Here's how the part is built. I have some questions about the finished solid (model axes, mm). Give positions to 0.01 mm unless a question says otherwise; leave off trailing zeros. Order: outer loops, then holes, each group sorted by start corner. A loop starts at its lowest first (then second) coordinate and runs counter-clockwise, first axis right, second up. Notation, with made-up numbers: (67.5, 44.25) - (126.5, 44.25) arc R11 ccw to (126.5, 63.25) - close; hole circle Ø9 at (-4, -5). An arc over 180 degrees is marked (long way). One line per question, with ' | ' between items.
Autodesk Inventor part; units mm, degrees
ref_plane "YZ Plane" through (0, 0, 0) normal (1, 0, 0) x (0, 1, 0)
ref_plane "XZ Plane" through (0, 0, 0) normal (0, 1, 0) x (-1, 0, 0)
ref_plane "XY Plane" through (0, 0, 0) normal (0, 0, 1) x (1, 0, 0)
sketch "スケッチ1" plane through (0, 0, 0) normal (0, 1, 0) x (-1, 0, 0)
  line L0 (0, 0) -> (-287.5, 0)
  line L1 (-287.5, 0) -> (-287.5, -30)
  line L2 (-287.5, -30) -> (0, -30)
  line L3 (0, -30) -> (0, 0)
  arc A0 (-17.5, -30) -> (-17.5, 0) centre (-17.5, -15) ccw
  point P0 (-17.5, -12.5)
  dimension "d0" = 287.5
  dimension "d1" = 30
  dimension "d2" = 17.5
  dimension "d3" = 17.5
  dimension "d43" = 17.5
extrude "押し出し1" add sketch "スケッチ1" along normal blind 3 contours A0 L2 L1 L0
sketch "スケッチ2" plane through (0, 3, 0) normal (0, 1, 0) x (1, 0, 0)
  arc A0 (17.5, 30) -> (17.5, 0) centre (17.5, 15) ccw
  line L0 (287.5, 30) -> (17.5, 30)
  point P0 (0, 0)
  point P1 (2.5, 15)
hole "穴1" at (17.5, 3, -15) direction (0, -1, 0) diameter 16 end through all
sketch "スケッチ3" plane through (0, 3, 0) normal (0, 1, 0) x (1, 0, 0)
  line L0 (287.5, 0) -> (287.5, 30)
  arc A0 (17.5, 30) -> (17.5, 0) centre (17.5, 15) ccw construction
  line L1 (17.5, 15) -> (287.5, 15) construction
  line L2 (287.5, 0) -> (287.5, 30) construction
  point P0 (0, 0)
  point P1 (57.5, 15)
  point P2 (67.5, 15)
  point P3 (77.5, 15)
  point P4 (87.5, 15)
  point P5 (97.5, 15)
  point P6 (107.5, 15)
  point P7 (117.5, 15)
  point P8 (127.5, 15)
  point P9 (137.5, 15)
  point P10 (147.5, 15)
  point P11 (157.5, 15)
  point P12 (167.5, 15)
  point P13 (177.5, 15)
  point P14 (187.5, 15)
  point P15 (197.5, 15)
  point P16 (207.5, 15)
  point P17 (217.5, 15)
  point P18 (227.5, 15)
  point P19 (237.5, 15)
  point P20 (247.5, 15)
  point P21 (257.5, 15)
  point P22 (267.5, 15)
  point P23 (277.5, 15)
  dimension "d108" = 40
  dimension "d111" = 10
sketch "スケッチ8" plane through (0, 3, 0) normal (0, 1, 0) x (1, 0, 0)
  arc A0 (17.5, 30) -> (17.5, 0) centre (17.5, 15) ccw
  line L0 (2.5, 15) -> (40.1182, 15)
  line L1 (17.5, 0) -> (287.5, 0)
  line L2 (2.5, 15) -> (302.5, 15) construction
  circle A1 centre (17.5, 15) radius 8 construction
  point P0 (0, 0)
  point P1 (33.3, 4.5)
  point P2 (33.3, 25.5)
  dimension "d85" = 10.5
  dimension "d86" = 10.5
  dimension "d123" = 15.8
  dimension "d124" = 15.8
hole "穴6" [suppressed]
hole "穴7" at (57.5, 3, -15) at (67.5, 3, -15) at (77.5, 3, -15) at (87.5, 3, -15) at (97.5, 3, -15) at (107.5, 3, -15) at (117.5, 3, -15) at (127.5, 3, -15) at (137.5, 3, -15) at (147.5, 3, -15) at (157.5, 3, -15) at (167.5, 3, -15) at (177.5, 3, -15) at (187.5, 3, -15) at (197.5, 3, -15) at (207.5, 3, -15) at (217.5, 3, -15) at (227.5, 3, -15) at (237.5, 3, -15) at (247.5, 3, -15) at (257.5, 3, -15) at (267.5, 3, -15) at (277.5, 3, -15) direction (0, -1, 0) diameter 3.2 end through all
properties part number "shoulder1_lower_plate" material "アルミニウム 5052"
1) Thinking about a two-plate mould opening in Z: for faces 1 (the face through (22.368, 1.479, -21.349)), 2 (the face through (2.504, 1.479, -14.67)), 3 (the face through (147, 0, -18)), which applies, +Z half, -Z half, draft (parallel to the pull), parting line (faces both ways), or undercut?
Model answer:
face 1: undercut | face 2: parting line | face 3: draft
2) I want a section at A-A (y = 1.05). State how many separate pieces and enclosed holes the cut face has, plus the area to 3 significant figures.
Model answer:
separate pieces: 1 | enclosed holes: 24 | area: 8,070 mm2
3) I'm going to push a flat-ended pin straight in: P1, Ø2.5, axis at x = 227.5, z = -15, coming from the -Y side. Where does the tip first touch, or does it pass through?
Model answer:
P1: passes through
4) Please list where these lines run through material, in increasing order: L1, parallel to Z at x = 87.5, y = 1.4; L2, parallel to X at y = 2.35, z = -9; L3, parallel to Z at x = 21.5, y = 2.5.
Model answer:
L1: z = -30 to -16.6, -13.4 to 0 | L2: x = 3.75 to 12.21, 22.79 to 287.5 | L3: z = -30 to -21.93, -8.07 to 0
5) I want a section at B-B (x = 22). List the corners of the cut face in (y, z) for me, plus the area to 3 significant figures.
Model answer:
outline: (0, -30) - (3, -30) - (3, -21.61) - (0, -21.61) - close; (0, -8.39) - (3, -8.39) - (3, 0) - (0, 0) - close | area: 50.3 mm2
